Drawing for the job (mm, zero at the part's lowest x, y, z). Round coordinates to 2 decimals unless told otherwise and drop trailing zeros. Order: outer loops, then holes, each group sorted by start corner. A loop starts at its lowest first (then second) coordinate and runs counter-clockwise, first axis right, second up. Notation, with made-up numbers: (79, 51) - (105, 51) arc R17 ccw to (105, 63) - close; hole circle Ø5 at (10, -4). An arc over 180 degrees is marked (long way). Answer as a JSON object with one key per item and string values.
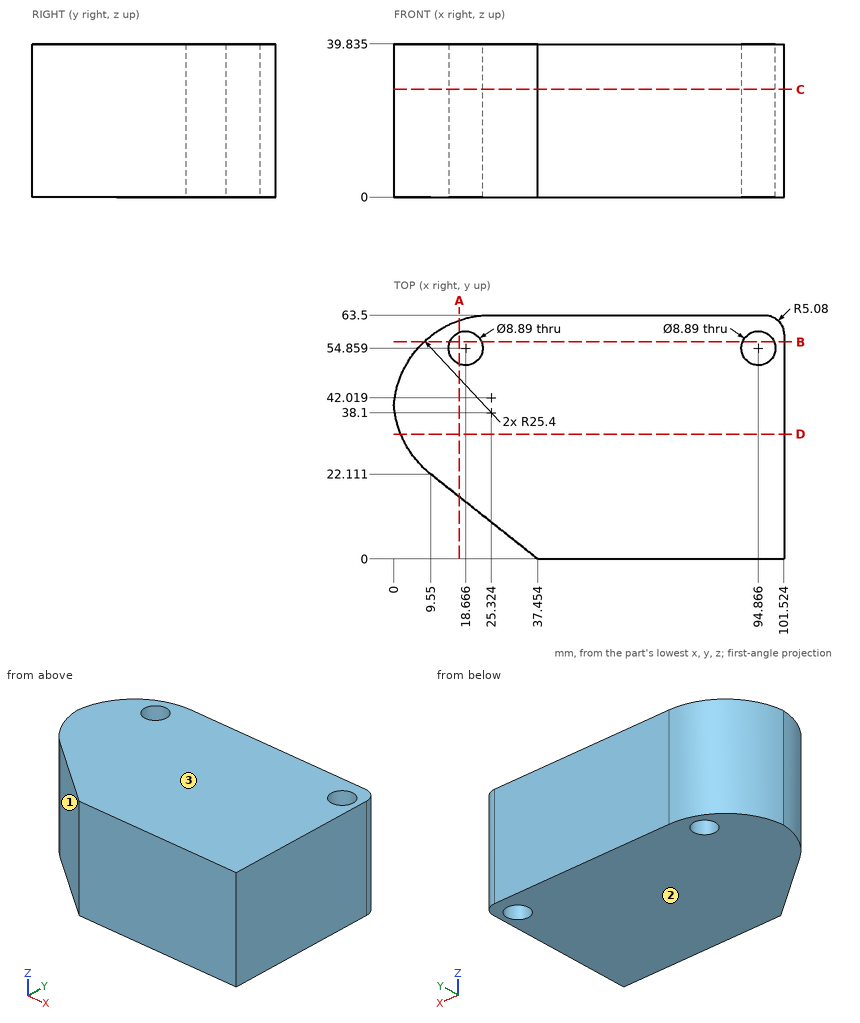
Item 1: Cut at C-C (z = 28). State how many separate pieces and enclosed holes the cut face has, plus the area to 3 significant figures.
Taken from the geometry:
{"separate pieces": "1", "enclosed holes": "2", "area": "5,600 mm2"}
Item 2: Two-plate mould, pull along Z, no slides. Class the marked faces 1, 2 and 3: pulls with the +Z half, pulls with the -Z half, needs draft (parallel to the pull), parting line crosses it, or undercut.
Taken from the geometry:
{"face 1": "needs draft", "face 2": "pulls with the -Z half", "face 3": "pulls with the +Z half"}
Item 3: Cut at B-B (y = 56.5). Write the cut outline in (x, z) (1 decimal).
Taken from the geometry:
{"outline": "(7.8, 0) - (14.5, 0) - (14.5, 39.8) - (7.8, 39.8) - close; (22.8, 0) - (90.7, 0) - (90.7, 39.8) - (22.8, 39.8) - close; (99, 0) - (101.5, 0) - (101.5, 39.8) - (99, 39.8) - close"}
Item 4: Probe L1, parallel to X at y = 54, z = 32.5 (1 decimal); L2, parallel to X at y = 56, z = 37 (1 decimal); L3, parallel to X at y = 23.5, z = 8.5 (1 decimal). List the from-to ranges inside material, lowest first. Write a range as from..to.
Taken from the geometry:
{"L1": "5.5..14.3, 23..90.5, 99.2..101.5", "L2": "7.3..14.4, 23..90.6, 99.2..101.5", "L3": "7.9..101.5"}
Item 5: Cut at D-D (y = 32.5). Write the cut outline in (x, z) (1 decimal), plus the area to 3 significant figures.
Taken from the geometry:
{"outline": "(1.8, 0) - (101.5, 0) - (101.5, 39.8) - (1.8, 39.8) - close", "area": "3,970 mm2"}
Item 6: Cut at A-A (x = 17). Write the cut outline in (y, z) (1 decimal).
Taken from the geometry:
{"outline": "(16.2, 0) - (50.7, 0) - (50.7, 39.8) - (16.2, 39.8) - close; (59, 0) - (62.1, 0) - (62.1, 39.8) - (59, 39.8) - close"}
Item 7: Drop flat-ended pins along their axis: P1, Ø3, axis at y = 15, z = 8.5, coming from the -X side; P2, Ø1, axis at y = 20, z = 22.5, coming from the -X side; P3, Ø2, axis at y = 49.5, z = 5.5, coming from the -X side. Give the stop position or say it passes through.
Taken from the geometry:
{"P1": "x = 16.63", "P2": "x = 11.58", "P3": "x = 2.15"}
